Read the model definition and answer for the solid it produces. Units are mm, in the model's axes. Face numbers are marked on the shaded views. Coordinates: 2 decimals unless noted, no trailing zeros. Answer as a JSON object with one key per item and string values. Group by question number.
(1) For a pull along Y with two mould halves and no side action, classify the marked faces 1 and 2 as +Y half, -Y half, draft (parallel to the pull), parting line (faces both ways), or undercut.
(2) Flat-ended cylindrical pins translate along their axes: P1, Ø12, axis at x = -47.5, z = -14.5, coming from the -Y side; P2, Ø6, axis at x = -31, z = -30, coming from the +Y side; P3, Ø1, axis at y = -4.5, z = -26.5, coming from the +X side. Find the tip coordinate at first contact, or state that the pin passes through.
(3) Straight lines are drawn through the part: L1, parallel to Y at x = 7.5, z = -21; L2, parallel to Y at x = 25, z = -22 (3 decimals); L3, parallel to Z at x = 4, y = 17.5. For each, find the intervals that lie inside material, in ascending order.
from build123d import *

# Parameters (mm, degrees)
FILLET1_R = 10


with BuildPart() as part:
    # Sketch3 → Loft1 section 0
    with BuildSketch(Plane.XY):
        with BuildLine():
            Line((62.5, -35), (-62.5, -35))
            Line((-62.5, -35), (-62.5, 35))
            Line((-62.5, 35), (62.5, 35))
            Line((62.5, 35), (62.5, -35))
        make_face()
    # Sketch4 → Loft1 section 1
    with BuildSketch(Plane.XY.offset(-40)):
        with BuildLine():
            Line((82.5, -47.5), (-82.5, -47.5))
            Line((-82.5, -47.5), (-82.5, 47.5))
            Line((-82.5, 47.5), (82.5, 47.5))
            Line((82.5, 47.5), (82.5, -47.5))
        make_face()
    loft()

    # Sketch7 → Cut-Loft2 section 0
    with BuildSketch(Plane.XY.offset(-40)):
        with BuildLine():
            Line((77.5, -42.5), (-77.5, -42.5))
            Line((-77.5, -42.5), (-77.5, 42.5))
            Line((-77.5, 42.5), (77.5, 42.5))
            Line((77.5, 42.5), (77.5, -42.5))
        make_face()
    # Sketch5 → Cut-Loft2 section 1
    with BuildSketch(Plane.XY.offset(-20)):
        with BuildLine():
            Line((22.5, -12.5), (-22.5, -12.5))
            Line((-22.5, -12.5), (-22.5, 12.5))
            Line((-22.5, 12.5), (22.5, 12.5))
            Line((22.5, 12.5), (22.5, -12.5))
        make_face()
    loft(mode=Mode.SUBTRACT)

    # Fillet1
    fillet1_edges = [part.edges().sort_by_distance(p)[0] for p in [
        (-72.5, -41.25, -20),
        (-72.5, 41.25, -20),
        (72.5, -41.25, -20),
        (72.5, 41.25, -20),
    ]]
    fillet(fillet1_edges, radius=FILLET1_R)


solid = part.part
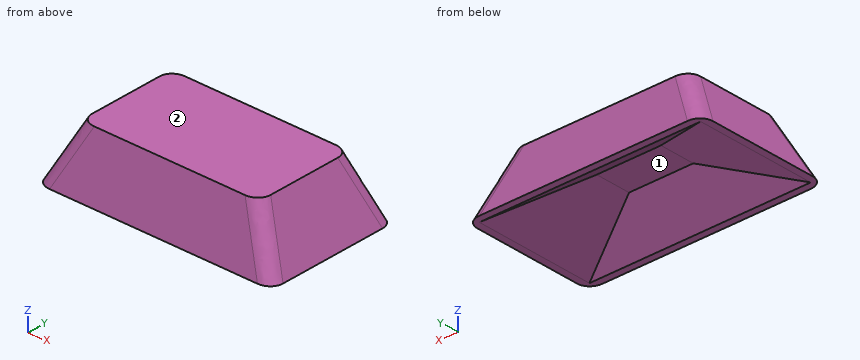
Results below:
{
 "1": {"face 1": "undercut", "face 2": "draft"},
 "2": {"P1": "stops at y = -41.41", "P2": "stops at y = 45.31", "P3": "stops at x = 76"},
 "3": {"L1": "y = -41.56 to -14, 14 to 41.56", "L2": "y = -41.875 to -15.5, 15.5 to 41.875", "L3": "z = -23.33 to 0"}
}
